Input: part model. Units: mm. Frame: model coordinates. A direction names the side the tool comes from. Coordinates: 2 decimals unless noted, no trailing zeros. Loops run counter-clockwise (first coordinate to the right, second up) from the corner with the lowest first, then second, coordinate; pieces in that order, holes last. Notation, with made-up numbers: (49, 45) - (75, 45) arc R22 ccw to (75, 55) - close; hole circle Ø10 at (-13, -10.5). An arc over 180 degrees is marked (long way). Use one line per item in the form item = value.
Autodesk Inventor part; units mm, degrees
ref_plane "YZ Plane" through (0, 0, 0) normal (1, 0, 0) x (0, 1, 0)
ref_plane "XZ Plane" through (0, 0, 0) normal (0, 1, 0) x (-1, 0, 0)
ref_plane "XY Plane" through (0, 0, 0) normal (0, 0, 1) x (1, 0, 0)
sketch "Sketch1" plane through (0, 0, 0) normal (0, 1, 0) x (-1, 0, 0)
  line L0 (0, 9.2388) -> (8.001, 4.6194)
  line L1 (8.001, 4.6194) -> (8.001, -4.6194)
  line L2 (8.001, -4.6194) -> (0, -9.2388)
  line L3 (10.541, -6.0858) -> (0, -12.1717)
  line L4 (0, 12.1717) -> (10.541, 6.0858)
  line L5 (10.541, 6.0858) -> (10.541, -6.0858)
  line L6 (0, 12.1717) -> (0, 9.2388)
  line L7 (0, -9.2388) -> (0, -12.1717)
  point P0 (0, 0)
  point P1 (0, 0)
  point P2 (0, 0)
  point P3 (0, 0)
  dimension "d5" = 2.54
extrude "Extrusion1" add sketch "Sketch1" along normal blind 7.62
sketch "Sketch2" plane through (-10.541, 0, -6.0858) normal (-1, 0, 0) x (0, 0, 1)
  circle A0 centre (6.0833, 3.81) radius 2.54
  line L0 (0, 0) -> (12.1717, 0)
  line L1 (12.1717, 0) -> (12.1717, 7.62)
  line L2 (0, 0) -> (0, 7.62)
  point P0 (6.0858, 0)
  dimension "d8" = 5.08
  dimension "d9" = 3.81
  dimension "d10" = 12.1717
  dimension "d11" = 6.0833
extrude "Extrusion2" cut sketch "Sketch2" against normal through all
properties part number "GearboxDogHolder"
Q1. Cut plane B-B, the plane x = -6. Return loops of the section in (y, z), then the cut area to 3 significant figures.
Check values:
outline = (0, -8.71) - (7.62, -8.71) - (7.62, -5.77) - (0, -5.77) - close; (0, 5.77) - (7.62, 5.77) - (7.62, 8.71) - (0, 8.71) - close
area = 44.7 mm²
Q2. Ray query, line 1 along X through (y, z) = (0.5, 3.25); line 2 along Y through (x, z) = (-9, -1); line 3 along Z through (x, y) = (-3, 1). Return the intervals inside material, ascending. Write a range as [from, to].
Check values:
line_1 = [-10.54, -8]
line_2 = [0, 1.47], [6.15, 7.62]
line_3 = [-10.44, -7.51], [7.51, 10.44]
Q3. Cut plane D-D, the plane y = 0.75. Return loops of the section in (x, z).
Check values:
outline = (-10.54, -6.09) - (0, -12.17) - (0, -9.24) - (-8, -4.62) - (-8, 4.62) - (0, 9.24) - (0, 12.17) - (-10.54, 6.09) - close
Q4. Pull-direction query (Z, two-part tool) for faces 3 (the flat face through (-5.34, 3.76, -9.09)), 4 (the flat face through (-5.2, 3.76, 9.17)), 5 (the cylindrical face through (-9.29, 6.33, -0.33)); classes: pulls with the +Z half, pulls with the -Z half, needs draft (parallel to the pull), parting line crosses it, or undercut.
Check values:
face_3 = pulls with the -Z half
face_4 = pulls with the +Z half
face_5 = undercut
Q5. Cut plane C-C, the plane z = -0.75. Return loops of the section in (x, y).
Check values:
outline = (-10.54, 0) - (-8, 0) - (-8, 1.38) - (-10.54, 1.38) - close; (-10.54, 6.24) - (-8, 6.24) - (-8, 7.62) - (-10.54, 7.62) - close
Q6. First-contact query: P1, Ø1, axis at x = -9.5, y = 6.5, coming from the -Z side; P2, Ø2, axis at y = 4.5, z = 1, coming from the +X side; P3, Ø3, axis at x = -7, y = 3, coming from the +Z side; P4, Ø3, axis at x = -2.5, z = -9, coming from the -Y side. Flat tips, straight axial feed; report the tip coordinate or a pass-through.
Check values:
P1 = -6.98
P2 = through
P3 = 9
P4 = 0
Q7. Cut plane A-A, the plane y = 3.81. Return loops of the section in (x, z).
Check values:
outline = (-10.54, -6.09) - (0, -12.17) - (0, -9.24) - (-8, -4.62) - (-8, -2.54) - (-10.54, -2.54) - close; (-10.54, 2.54) - (-8, 2.54) - (-8, 4.62) - (0, 9.24) - (0, 12.17) - (-10.54, 6.09) - close
Q8. Set-up query: faces 1 (the flat face through (-10.541, 1, 0)), 2 (the flat face through (-3.944, 3.757, 6.961)). Return all of +Z, -Z, +X, -X, +Y, -Y with unobstructed straight access to the full face (end or side cutting, diameter ignored); none if empty.
Check values:
face_1 = +Z, -Z, -X, +Y, -Y
face_2 = +X, +Y, -Y
